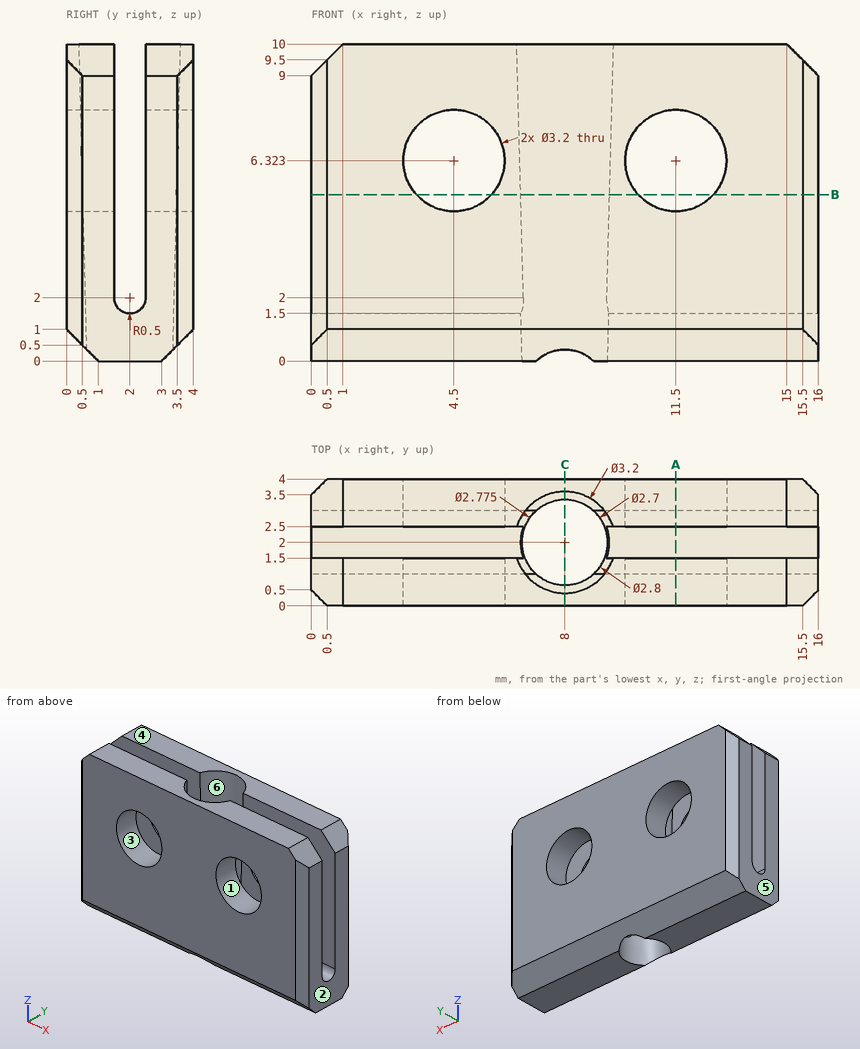
Verification items for this drawing (mm, ordinates from the low corner). A direction names the side the tool comes from. Give positions to 0.01 mm unless a question says otherwise; leave off trailing zeros. Loops run counter-clockwise (first coordinate to the right, second up) from the corner with the lowest first, then second, coordinate; pieces in that order, holes last.
1. Release check for a two-part mould opening along X. For the marked faces 1, 2, 3 and 4 record: +X half, -X half, draft (parallel to the pull), parting line (faces both ways), or undercut.
Derived:
face 1: undercut
face 2: +X half
face 3: undercut
face 4: draft
2. Cross-section at B-B on z = 5.25. Count the separate pieces of the cut face and the enclosed holes in it.
Derived:
separate pieces: 6
enclosed holes: 0
3. Cross-section at A-A on x = 11.5. Record the cut outline in (y, z).
Derived:
outline: (0, 1) - (1, 0) - (3, 0) - (4, 1) - (4, 4.72) - (2.5, 4.72) - (2.5, 2) arc R0.5 cw to (1.5, 2) - (1.5, 4.72) - (0, 4.72) - close; (0, 7.92) - (1.5, 7.92) - (1.5, 10) - (0, 10) - close; (2.5, 7.92) - (4, 7.92) - (4, 10) - (2.5, 10) - close
4. Material ranges on probe 1 along Z at (x, y) = (4.5, 1.05); probe 2 along Y at (x, z) = (13, 8.75); probe 3 along Z at (x, y) = (4.5, 0.5), recorded low to high.
Derived:
probe 1: z = 0 to 4.72, 7.92 to 10
probe 2: y = 0 to 1.5, 2.5 to 4
probe 3: z = 0.5 to 4.72, 7.92 to 10
5. Cross-section at C-C on x = 8. Record the cut outline in (y, z).
Derived:
outline: (0, 1) - (0.64, 0.36) - (0.4, 10) - (0, 10) - close; (3.36, 0.36) - (4, 1) - (4, 10) - (3.6, 10) - close
6. Tool access check on the marked faces 5 and 6. Record the directions out of +Z, -Z, +X, -X, +Y, -Y that give a thin tool (end or side, any length) a straight path to the whole face; none if there is none.
Derived:
face 5: +Z, -Z, -X, +Y, -Y
face 6: +Z
7. Go/stop test with a flat-tipped pin: P1, Ø3.5, axis at x = 11.5, z = 6.32, coming from the -Y side. Record where the tip stops, or that it passes through.
Derived:
P1: stops at y = 0
